from build123d import *

# Parameters (mm, degrees)
F1_DEPTH    = 4.064
F2_DEPTH    = 2.794
F3_R        = 3.6792614691
F4_T1_DEPTH = 129.0096523961


# Not quite as in the source:
# - a fillet or chamfer that OpenCascade refuses, or shapes differently, is made with other operations: its cross-section is extruded or revolved along the edge and cut away or added


with BuildPart() as f1:
    # F0 (on Right) → F1 (new body)
    with BuildSketch(Plane.YZ):
        Polygon((72.7801844478, 0), (0, 76.3147622347), (0, 0), align=None)
    extrude(amount=F1_DEPTH)

    # F2 (add): a face of the model
    f2_faces = [f1.faces().sort_by_distance(p)[0] for p in [
        (0, 24.2600614826, 25.4382540782),
    ]]
    extrude(f2_faces, amount=F2_DEPTH)

    # F3
    f3_edges = [f1.edges().sort_by_distance(p)[0] for p in [
        (-2.794, 36.390092, 38.157381),
    ]]
    fillet(f3_edges, radius=F3_R)

    # F4: fillet of radius 5.08 on 1 edges, made by hand

    # F4_s2 → F4_t1 (cut)
    with BuildSketch(Plane(origin=(0, 42.7935550314, -44.8718288113), x_dir=(1, 0, 0), z_dir=(0, -0.6901495666, 0.7236667574))):
        with BuildLine():
            ThreePointArc((0.8852614691, 52.6686000807), (3.1949861234, 50.7992812188), (4.064, 47.9578034574))
            Line((4.064, 47.9578034574), (4.064, 52.6686000807))
            Line((4.064, 52.6686000807), (0.8852614691, 52.6686000807))
        make_face()
    extrude(amount=F4_T1_DEPTH, mode=Mode.SUBTRACT)


solid = f1.part
Model file for the job. Use its own axes, mm. Give positions to 0.01 mm unless a question says otherwise; leave off trailing zeros. Order: outer loops, then holes, each group sorted by start corner. A loop starts at its lowest first (then second) coordinate and runs counter-clockwise, first axis right, second up. Notation, with made-up numbers: (71, 37.5) - (84, 37.5) arc R23 cw to (84, 58.5) - close; hole circle Ø8 at (63.25, -4.5). An arc over 180 degrees is marked (long way). Write item = value, one per line. Start each with the question number.
1. Probe line 1 along Z through (x, y) = (-0.75, 41); line 2 along Z through (x, y) = (3, 25); line 3 along Y through (x, z) = (0.5, 59). List the from-to ranges inside material, lowest first.
2. Drop a flat-ended pin along its axis: P1, Ø3, axis at x = 1.5, z = 34.5, coming from the +Y side. Give the stop position or say it passes through.
3. Cut at A-A, the plane x = 2.5. List the corners of the cut face in (y, z), and give its area (3 significant figures).
4. Cut at B-B, the plane x = -1.5. List the corners of the cut face in (y, z), and give its area (3 significant figures).
5. Two-plate mould, pull along X, no slides. Class faces 1 (the flat face through (1, 0, 39)), 2 (the flat face through (-2.794, 18, 20)), 3 (the cylindrical face through (3.17, 35.57, 36.36)): pulls with the +X half, pulls with the -X half, needs draft (parallel to the pull), parting line crosses it, or undercut.
Taken from the geometry:
q1.line_1 = 0 to 32.77
q1.line_2 = 0 to 47.78
q1.line_3 = 0 to 16.48
q2.P1 = 41.18
q3.outline = (0, 0) - (71.34, 0) - (0, 74.8) - close
q3.area = 2,670 mm²
q4.outline = (0, 0) - (71.57, 0) - (0, 75.04) - close
q4.area = 2,690 mm²
q5.face_1 = needs draft
q5.face_2 = pulls with the -X half
q5.face_3 = pulls with the +X half
